```python
from build123d import *

# Parameters (mm, degrees)
F0_W     = 250
F0_H     = 20
F1_DEPTH = 20
F2_W     = 20
F2_H     = 20
F3_DEPTH = 10
F4_W     = 100
F4_H     = 20
F5_DEPTH = 10


with BuildPart() as f1:
    # F0 (on Top) → F1 (new body)
    with BuildSketch(Plane.XY):
        Rectangle(F0_W, F0_H)
    extrude(amount=F1_DEPTH)

    # F2 (on face) → F3 (cut)
    with BuildSketch(Plane.XZ.offset(10)):
        with Locations((85, 10)):
            Rectangle(F2_W, F2_H)
    extrude(amount=-F3_DEPTH, mode=Mode.SUBTRACT)

    # F4 (on face) → F5 (cut)
    with BuildSketch(Plane.XY.offset(20)):
        with Locations((-45, 0)):
            Rectangle(F4_W, F4_H)
    extrude(amount=-F5_DEPTH, mode=Mode.SUBTRACT)


solid = f1.part
```
Can you work these out from the model? Positions are in its coordinate system, mm. A direction names the side the tool comes from. Coordinates: 2 decimals unless noted, no trailing zeros. Order: outer loops, then holes, each group sorted by start corner. A loop starts at its lowest first (then second) coordinate and runs counter-clockwise, first axis right, second up. Notation, with made-up numbers: (62.5, -24.75) -> (85.5, -24.75) arc R21 cw to (85.5, -12.75) -> close; hole circle Ø8 at (-37.75, 16.25). An arc over 180 degrees is marked (long way). Write each question's results on one line, items separated by ' | '.
Item 1: I want a section at B-B, the plane y = -4.25. Write out the boundary of the cut face in (x, z).
Results are:
outline: (-125, 0) -> (75, 0) -> (75, 20) -> (5, 20) -> (5, 10) -> (-95, 10) -> (-95, 20) -> (-125, 20) -> close; (95, 0) -> (125, 0) -> (125, 20) -> (95, 20) -> close
Item 2: I want a section at A-A, the plane z = 15.5. Write out the boundary of the cut face in (x, y).
Results are:
outline: (-125, -10) -> (-95, -10) -> (-95, 10) -> (-125, 10) -> close; (5, -10) -> (75, -10) -> (75, 0) -> (95, 0) -> (95, -10) -> (125, -10) -> (125, 10) -> (5, 10) -> close
Item 3: Which directions (+Z, -Z, +X, -X, +Y, -Y) give clear straight access to the entire face, cutting with the end or side of a thin tool? Please do faces 1 (the face through (-46, 0, 10)), 2 (the face through (75, -5, 10)), 3 (the face through (-125, 0, 10)).
Results are:
face 1: +Z, +Y, -Y | face 2: +Z, -Z, -Y | face 3: +Z, -Z, -X, +Y, -Y
Item 4: I want a section at C-C, the plane y = 6. Write out the boundary of the cut face in (x, z), then the cut area to 3 significant figures.
Results are:
outline: (-125, 0) -> (125, 0) -> (125, 20) -> (5, 20) -> (5, 10) -> (-95, 10) -> (-95, 20) -> (-125, 20) -> close | area: 4,000 mm²
Item 5: I want a section at D-D, the plane z = 4.5. Write out the boundary of the cut face in (x, y).
Results are:
outline: (-125, -10) -> (75, -10) -> (75, 0) -> (95, 0) -> (95, -10) -> (125, -10) -> (125, 10) -> (-125, 10) -> close
Item 6: If I drill on line 1 along X through (y, z) = (-7.5, 17.5); line 2 along X through (y, z) = (5, 17.5); line 3 along X through (y, z) = (-5.75, 5.5), over which ranges is the centre line in solid material (lowest first)?
Results are:
line 1: -125 to -95, 5 to 75, 95 to 125 | line 2: -125 to -95, 5 to 125 | line 3: -125 to 75, 95 to 125
